Read the model definition and answer for the solid it produces. Units are mm, in the model's axes. Face numbers are marked on the shaded views. Coordinates: 2 decimals unless noted, no trailing zeros. Loops run counter-clockwise (first coordinate to the right, second up) from the corner with the lowest first, then second, coordinate; pieces in that order, holes last.
Autodesk Inventor part; units mm, degrees
ref_plane "Work Plane1" through (-26.022, 0, 0) normal (0, -0.866, -0.5) x (1, 0, 0)
ref_plane "YZ Plane" through (0, 0, 0) normal (1, 0, 0) x (0, 1, 0)
ref_plane "XZ Plane" through (0, 0, 0) normal (0, 1, 0) x (-1, 0, 0)
sketch "Sketch1" plane through (0, 0, 0) normal (1, 0, 0) x (0, 1, 0)
  line L0 (-12.1244, 0) -> (-6.0622, 10.5)
  line L1 (-6.0622, 10.5) -> (6.0622, 10.5)
  line L2 (6.0622, 10.5) -> (12.1244, 0)
  line L3 (12.1244, 0) -> (6.0622, -10.5)
  line L4 (6.0622, -10.5) -> (-6.0622, -10.5)
  line L5 (-6.0622, -10.5) -> (-12.1244, 0)
  point P0 (0, 0)
  point P1 (0, 0)
  dimension "d0" = 24.2487
extrude "Body" add sketch "Sketch1" along normal blind 7
sketch "Sketch2" plane through (0, 0, 0) normal (0, 0, 1) x (1, 0, 0)
  line L0 (0, 6.0622) -> (0, 12.1244)
  line L1 (0, 12.1244) -> (7, 12.1244)
  line L2 (7, 6.0622) -> (7, 12.1244)
  line L3 (-1.4, 0) -> (8.4, 0)
  line L4 (1.3304, 12.1244) -> (0, 9.82)
  line L5 (5.6696, 12.1244) -> (7, 9.82)
  dimension "d3" = 30
  dimension "d4" = 30
  dimension "d5" = 19.64
  dimension "d6" = 19.64
revolve "Chamfer1" cut sketch "Sketch2" angle 360 about axis through (-10, 0, 0) along (1, 0, 0)
sketch "Sketch3" plane through (7, 0, 0) normal (1, 0, 0) x (0, 0, -1)
  arc A0 (-0.625, -1.0825) -> (0.625, -1.0825) centre (0, 0) ccw
hole "Thread" at (7, 0, 0) direction (-1, 0, 0) diameter 12.376 end through all
chamfer "Chamfer2" distance 0.8119 angle 30 1 edges at (7, 0, 6.188) measured on face at (7, 8.4992, -1.032)
chamfer "Chamfer3" distance 0.8119 angle 30 1 edges at (0, 0, 6.188) measured on face at (0, 8.4992, -1.032)
ref_plane "Work Plane1" through (-26.022, 0, 0) normal (0, -0.866, -0.5) x (1, 0, 0)
equation "\"d0\" = 1.1547 * SW"
equation "\"d1\" = KOH"
equation "\"d3\" = ANG1"
equation "\"d4\" = ANG2"
equation "\"d5\" = SW0"
equation "\"d6\" = SW01"
equation "\"d8\" = -0.5 * GD1 + 0.5 * NND"
equation "\"d40\" = -0.5 * GD1 + 0.5 * NND"
equation "\"d10\" = -0.5 * GD1 + 0.5 * NND"
equation "\"d41\" = -0.5 * GD1 + 0.5 * NND"
equation "\"ANG1\" = 30deg"
equation "\"ANG2\" = 30deg"
equation "\"NND\" = 14"
equation "\"KOH\" = 7"
equation "\"SW\" = 21"
equation "\"SW0\" = 19.64"
equation "\"SW01\" = SW0"
equation "\"GUL\" = 0.541266 * PTC"
equation "\"THREADDIA\" = 14"
equation "\"TOA\" = 30deg"
equation "\"PTC\" = 1.5"
equation "\"E0\" = 23.36"
equation "\"GAL\" = 0.541266 * PTC"
properties part number "ISO 8675 - M14 x 1.5" material "Stainless Steel, 440C"
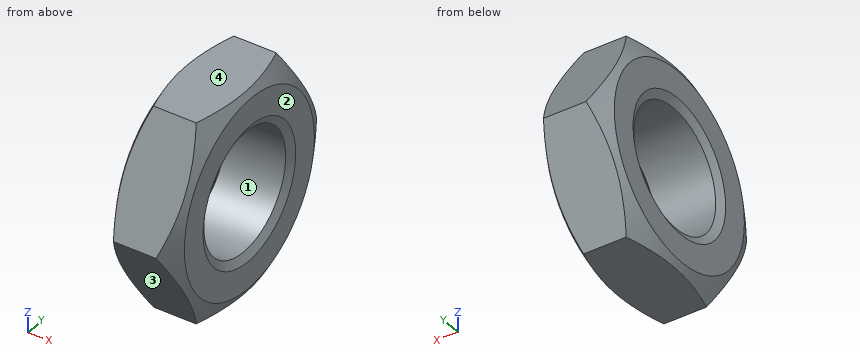
Q1. Straight lines are drawn through the part: probe 1 along Z at (x, y) = (5.25, 0); probe 2 along Y at (x, z) = (2.75, -3.25); probe 3 along Y at (x, z) = (1, -1.25). For each, find the intervals that lie inside material, in ascending order.
Findings below:
probe 1: z = -10.5 to -6.19, 6.19 to 10.5
probe 2: y = -10.25 to -5.27, 5.27 to 10.25
probe 3: y = -11.4 to -6.06, 6.06 to 11.4
Q2. Flat-ended cylindrical pins translate along their axes: pin 1 Ø1.5 at (x, z) = (2, 8.5) entering from -Y; pin 2 Ø4 at (x, z) = (4, -4.5) entering from +Y; pin 3 Ø2 at (x, y) = (3, -7.5) entering from -Z. Find the tip coordinate at first contact, or state that the pin passes through.
Findings below:
pin 1: stops at y = -7.65
pin 2: stops at y = 10.68
pin 3: stops at z = -9.74
Q3. A cutting plane is placed at A-A (y = 0). Give the vertices of the cut face in (x, z), then the cut area to 3 significant figures.
Findings below:
outline: (0, -9.82) - (0.39, -10.5) - (6.61, -10.5) - (7, -9.82) - (7, -7) - (6.53, -6.19) - (0.47, -6.19) - (0, -7) - close; (0, 7) - (0.47, 6.19) - (6.53, 6.19) - (7, 7) - (7, 9.82) - (6.61, 10.5) - (0.39, 10.5) - (0, 9.82) - close
area: 59.1 mm2
Q4. Determine the mould class of the marked faces 1, 2, 3 and 4 for opening direction Z: +Z half, -Z half, draft (parallel to the pull), parting line (faces both ways), or undercut.
Findings below:
face 1: undercut
face 2: draft
face 3: -Z half
face 4: +Z half
Q5. A cutting plane is placed at B-B (x = 2.75). Give the vertices of the cut face in (y, z), then the cut area to 3 significant figures.
Findings below:
outline: (-12.12, 0) - (-6.06, -10.5) - (6.06, -10.5) - (12.12, 0) - (6.06, 10.5) - (-6.06, 10.5) - close; hole circle Ø12.38 at (0, 0)
area: 262 mm2
